CAD build for the part. Positions are in the model's coordinates, mm. A direction names the side the tool comes from. Round coordinates to 2 decimals unless told otherwise and drop trailing zeros. Loops run counter-clockwise (first coordinate to the right, second up) from the corner with the lowest first, then second, coordinate; pieces in that order, holes last. Notation, with made-up numbers: (52, 50.25) -> (66, 50.25) arc R11 cw to (66, 54.25) -> close; hole circle Ø9 at (86.25, 26). An arc over 180 degrees is marked (long way). Answer as CSV lines item,"result".
```python
from build123d import *

# Parameters (mm, degrees)
F0_W     = 90
F0_H     = 50
F0_H_2   = 30
F0_R     = 1.55
F0_W_2   = 19
F0_H_3   = 3
F1_DEPTH = 4
F3_DEPTH = 4
F4_W     = 0.5
F4_H     = 20
F5_DEPTH = 0.5


with BuildPart() as f1:
    # F0 (on Front) → F1 (new body)
    with BuildSketch(Plane.XZ):
        Polygon((50.859297, 66.157015), (-49.140703, 66.157015), (-49.140703, -63.842985), (-9.140703, -63.842985), (-9.140703, -83.842985), (10.859297, -83.842985), (10.859297, -63.842985), (50.859297, -63.842985), align=None)
        with Locations((0.859297, -28.842985)):
            Rectangle(F0_W, F0_H, mode=Mode.SUBTRACT)
        with Locations((0.859297, 21.157015)):
            Rectangle(F0_W, F0_H_2, mode=Mode.SUBTRACT)
        with Locations((-26.640703, 41.357015)):
            Circle(F0_R, mode=Mode.SUBTRACT)
        with Locations((0.859297, 57.657015)):
            Rectangle(F0_W_2, F0_H_3, mode=Mode.SUBTRACT)
        with Locations((28.359297, 56.357015)):
            Circle(F0_R, mode=Mode.SUBTRACT)
    extrude(amount=F1_DEPTH)

    # F2 (on face) → F3 (join)
    with BuildSketch(Plane.XY.offset(6.157015)):
        with BuildLine():
            Line((-49.140703, 80), (-49.140703, 0))
            Line((-49.140703, 0), (-29.140703, 0))
            Line((-29.140703, 0), (-29.140703, 80))
            ThreePointArc((-29.140703, 80), (-30.605169, 83.535534), (-34.140703, 85))
            Line((-34.140703, 85), (-44.140703, 85))
            ThreePointArc((-44.140703, 85), (-47.676237, 83.535534), (-49.140703, 80))
        make_face()
        Polygon((-46.854805, 37), (-43.390703, 39), (-39.926602, 37), (-39.926602, 33), (-43.390703, 31), (-46.854805, 33), align=None, mode=Mode.SUBTRACT)
        with BuildLine():
            Line((30.859297, 80), (30.859297, 0))
            Line((30.859297, 0), (50.859297, 0))
            Line((50.859297, 0), (50.859297, 80))
            ThreePointArc((50.859297, 80), (49.394831, 83.535534), (45.859297, 85))
            Line((45.859297, 85), (35.859297, 85))
            ThreePointArc((35.859297, 85), (32.323763, 83.535534), (30.859297, 80))
        make_face()
        Polygon((45.109297, 39), (48.573398, 37), (48.573398, 33), (45.109297, 31), (41.645195, 33), (41.645195, 37), align=None, mode=Mode.SUBTRACT)
    extrude(amount=-F3_DEPTH)

    # F4 (on face) → F5 (cut)
    with BuildSketch(Plane(origin=(0, 0, 0), x_dir=(-1, 0, 0), z_dir=(0, 1, 0))):
        with Locations((-0.859297, -73.842985)):
            Rectangle(F4_W, F4_H)
    extrude(amount=-F5_DEPTH, mode=Mode.SUBTRACT)


solid = f1.part
```
Q1. Tool access for faces 1 (the flat face through (-41.634, 32.014, 4.185)), 2 (the cylindrical face through (32.36, 83.57, 4.19)), 3 (the flat face through (0, -2, -53.843)), 4 (the flat face through (31, -2, -63.843)), 5 (the flat face through (0, 0, 50)): list every direction of +Z, -Z, +X, -X, +Y, -Y with a clear straight run to the whole face (end or side of a thin tool).
Results:
face 1,"+Z, -Z"
face 2,"+Z, -Z, +Y"
face 3,"+Y, -Y"
face 4,"-Z, +X, +Y, -Y"
face 5,"+Z, +X, -X, +Y"
Q2. Slice it at B-B, the plane z = -18. Give the cut face in (x, y), and give its area (3 significant figures).
Results:
outline,"(-49.14, -4) -> (-44.14, -4) -> (-44.14, 0) -> (-49.14, 0) -> close; (45.86, -4) -> (50.86, -4) -> (50.86, 0) -> (45.86, 0) -> close"
area,"40.0 mm2"
Q3. Drop flat-ended pins along their axis: pin 1 Ø6 at (x, z) = (31.5, 48) entering from +Y; pin 2 Ø1.2 at (x, y) = (-17, -1.5) entering from -Z; pin 3 Ø22 at (x, y) = (-43, 55.5) entering from -Z. Give the stop position or say it passes through.
Results:
pin 1,"y = 0"
pin 2,"z = -63.84"
pin 3,"z = 2.16"
Q4. Two-plate mould, pull along Y, no slides. Class faces 6 (the flat face through (-44.141, -2, 21)), 7 (the cylindrical face through (-47.64, 83.57, 4.19)), 8 (the flat face through (46.866, 32.014, 4.185)): pulls with the +Y half, pulls with the -Y half, needs draft (parallel to the pull), parting line crosses it, or undercut.
Results:
face 6,"needs draft"
face 7,"pulls with the +Y half"
face 8,"undercut"
Q5. Slice it at C-C, the plane x = -13. Give the cut face in (y, z), and give its area (3 significant figures).
Results:
outline,"(-4, -63.84) -> (0, -63.84) -> (0, -53.84) -> (-4, -53.84) -> close; (-4, -3.84) -> (0, -3.84) -> (0, 6.16) -> (-4, 6.16) -> close; (-4, 36.16) -> (0, 36.16) -> (0, 66.16) -> (-4, 66.16) -> close"
area,"200 mm2"
Q6. Slice it at A-A, the plane y = 42. Give the cut face in (x, z), and give its area (3 significant figures).
Results:
outline,"(-49.14, 2.16) -> (-29.14, 2.16) -> (-29.14, 6.16) -> (-49.14, 6.16) -> close; (30.86, 2.16) -> (50.86, 2.16) -> (50.86, 6.16) -> (30.86, 6.16) -> close"
area,"160 mm2"
Q7. Slice it at D-D, the plane x = 3. Give the cut face in (y, z), and give its area (3 significant figures).
Results:
outline,"(-4, -83.84) -> (0, -83.84) -> (0, -53.84) -> (-4, -53.84) -> close; (-4, -3.84) -> (0, -3.84) -> (0, 6.16) -> (-4, 6.16) -> close; (-4, 36.16) -> (0, 36.16) -> (0, 56.16) -> (-4, 56.16) -> close; (-4, 59.16) -> (0, 59.16) -> (0, 66.16) -> (-4, 66.16) -> close"
area,"268 mm2"
Q8. Probe L1, parallel to Y at x = 6.5, z = -74; L2, parallel to Z at x = 40, y = 4. List the from-to ranges inside material, lowest first. Write a range as [from, to].
Results:
L1,"[-4, 0]"
L2,"[2.16, 6.16]"
